Autodesk Fusion 360 part; units mm, degrees
sketch "Sketch1" plane through (0, 0, 0) normal (1, 0, 0) x (0, 1, 0)
  line L0 (0, 0) -> (180, 0)
  line L1 (180, 0) -> (180, 25)
  line L2 (180, 25) -> (170, 25)
  line L3 (170, 25) -> (170, 70)
  line L4 (170, 70) -> (180, 70)
  line L5 (180, 70) -> (180, 105)
  line L6 (180, 105) -> (170, 105)
  line L7 (170, 105) -> (0, 105)
  line L8 (0, 105) -> (0, 70)
  line L9 (0, 70) -> (10, 70)
  line L10 (10, 70) -> (10, 25)
  line L11 (10, 25) -> (0, 25)
  line L12 (0, 25) -> (0, 0)
  line L13 (0, 0) -> (50, 0)
  line L14 (50, 0) -> (50, 7)
  line L15 (50, 7) -> (0, 7)
  line L16 (0, 7) -> (0, 0)
  line L17 (180, 0) -> (130, 0)
  line L18 (130, 0) -> (130, 7)
  line L19 (130, 7) -> (180, 7)
  line L20 (180, 7) -> (180, 0)
  dimension "d1" = 180
  dimension "d2" = 10
  dimension "d4" = 25
  dimension "d5" = 105
  dimension "d6" = 10
  dimension "d20" = 35
  dimension "d22" = 7
  dimension "d23" = 50
  dimension "d26" = 80
extrude "Extrude1" add sketch "Sketch1" along normal blind 5 contours L0 L1 L2 L3 L4 L5 L6 L7 L8 L9 L10 L11 L12 L14 L15 L18 L19
sketch "Sketch2" plane through (5, 0, 0) normal (1, 0, 0) x (0, 1, 0)
  line L0 (0, 25) -> (0, 0)
  line L1 (0, 0) -> (180, 0)
  line L2 (180, 0) -> (180, 25)
  line L3 (180, 25) -> (170, 25)
  line L4 (170, 25) -> (170, 70)
  line L5 (170, 70) -> (180, 70)
  line L6 (180, 70) -> (180, 105)
  line L7 (180, 105) -> (0, 105)
  line L8 (0, 105) -> (0, 70)
  line L9 (0, 70) -> (10, 70)
  line L10 (10, 70) -> (10, 25)
  line L11 (10, 25) -> (0, 25)
  line L12 (134.6138, 69.8664) -> (134.6138, 24.8664)
  arc A0 (134.6138, 24.8664) -> (154.6138, 24.8664) centre (144.6138, 24.8664) ccw
  line L13 (154.6138, 24.8664) -> (154.6138, 69.8664)
  arc A1 (154.6138, 69.8664) -> (134.6138, 69.8664) centre (144.6138, 69.8664) ccw
  line L14 (144.6138, 69.8664) -> (144.6138, 24.8664) construction
  line L15 (50, 96.5) -> (130, 96.5)
  line L16 (130, 96.5) -> (130, 90)
  line L17 (130, 90) -> (50, 90)
  line L18 (50, 90) -> (50, 96.5)
  dimension "d9" = 20
  dimension "d15" = 90
  dimension "d16" = 6.5
  dimension "d17" = 80
  dimension "d18" = 50
  dimension "d25" = 45
extrude "Extrude2" cut sketch "Sketch2" against normal through all contours L12 A0 L13 A1
pattern_linear "R-Pattern1" count 1 spacing 0 along (0, 0, -1) count 5 spacing 27.5 along (0, -1, 0) of "Extrude2"
extrude "Extrude3" cut sketch "Sketch2" against normal through all contours L15 L16 L17 L18
extrude "Extrude4" cut sketch "Sketch1" along normal through all contours L0 L12 L13 L14 L15 L16 | L0 L1 L17 L18 L19 L20
For this review, take the finished solid that the model builds, in its own axes (mm). A direction names the side the tool comes from. Round coordinates to 2 decimals unless told otherwise and drop trailing zeros. Order: outer loops, then holes, each group sorted by start corner. A loop starts at its lowest first (then second) coordinate and runs counter-clockwise, first axis right, second up. Notation, with made-up numbers: (33, -27) -> (58, -27) arc R25 ccw to (58, -6) -> close; hole circle Ø2 at (-16.75, 29). An arc over 180 degrees is marked (long way). Put each result on its own line as item: value.
Q1. Machinability: for faces 5 (the flat face through (2, 175, 70)), 6 (the flat face through (3, 50, 93)), 7 (the flat face through (2, 50, 3)), which of the approach directions +Z, -Z, +X, -X, +Y, -Y give a long, thin tool a straight path to every point of the face, cutting with its end or side? Answer none if there is none.
Check result:
face 5: +X, -X, +Y
face 6: +X, -X
face 7: -Z, +X, -X, -Y
Q2. Insertion check: pin 1 Ø2.5 at (x, z) = (2, 45) entering from +Y; pin 2 Ø2.5 at (x, z) = (3.5, 56.5) entering from -Y; pin 3 Ø1.5 at (x, y) = (2, 21) entering from -Z. Each pin has a flat end and moves straight along its axis. Give the tip position at first contact, or say it passes through.
Check result:
pin 1: y = 170
pin 2: y = 10
pin 3: z = 7
Q3. Add section A-A on z = 33. Write out the cut boundary in (x, y).
Check result:
outline: (0, 10) -> (5, 10) -> (5, 24.61) -> (0, 24.61) -> close; (0, 44.61) -> (5, 44.61) -> (5, 52.11) -> (0, 52.11) -> close; (0, 72.11) -> (5, 72.11) -> (5, 79.61) -> (0, 79.61) -> close; (0, 99.61) -> (5, 99.61) -> (5, 107.11) -> (0, 107.11) -> close; (0, 127.11) -> (5, 127.11) -> (5, 134.61) -> (0, 134.61) -> close; (0, 154.61) -> (5, 154.61) -> (5, 170) -> (0, 170) -> close
Q4. Add section C-C on z = 92. Write out the cut boundary in (x, y), plus the area to 3 significant figures.
Check result:
outline: (0, 0) -> (5, 0) -> (5, 50) -> (0, 50) -> close; (0, 130) -> (5, 130) -> (5, 180) -> (0, 180) -> close
area: 500 mm2
Q5. Mouldability with a two-part tool opening along Y and no side actions: class faces 1 (the flat face through (3, 107.114, 48)), 2 (the cylindrical face through (2.535, 34.834, 79.864)), 3 (the flat face through (2, 89, 0)), 4 (the flat face through (2, 170, 47)) as pulls with the +Y half, pulls with the -Y half, needs draft (parallel to the pull), parting line crosses it, or undercut.
Check result:
face 1: undercut
face 2: undercut
face 3: needs draft
face 4: pulls with the +Y half
Q6. Add section D-D on y = 149. Write out the cut boundary in (x, z).
Check result:
outline: (0, 7) -> (5, 7) -> (5, 15.88) -> (0, 15.88) -> close; (0, 78.85) -> (5, 78.85) -> (5, 105) -> (0, 105) -> close
Q7. For probe 1 along Y at (x, z) = (4.1, 52); probe 2 along Z at (x, y) = (3.95, 96); probe 3 along Y at (x, z) = (2.75, 74), list the stretches that pass through material, from the lowest coordinate up. Write a range as [from, to].
Check result:
probe 1: [10, 24.61], [44.61, 52.11], [72.11, 79.61], [99.61, 107.11], [127.11, 134.61], [154.61, 170]
probe 2: [0, 17.17], [77.56, 90], [96.5, 105]
probe 3: [0, 25.51], [43.72, 53.01], [71.22, 80.51], [98.72, 108.01], [126.22, 135.51], [153.72, 180]
Q8. Add section B-B on y = 86. Write out the cut boundary in (x, z), plus the area to 3 significant figures.
Check result:
outline: (0, 0) -> (5, 0) -> (5, 15.54) -> (0, 15.54) -> close; (0, 79.19) -> (5, 79.19) -> (5, 90) -> (0, 90) -> close; (0, 96.5) -> (5, 96.5) -> (5, 105) -> (0, 105) -> close
area: 174 mm2
